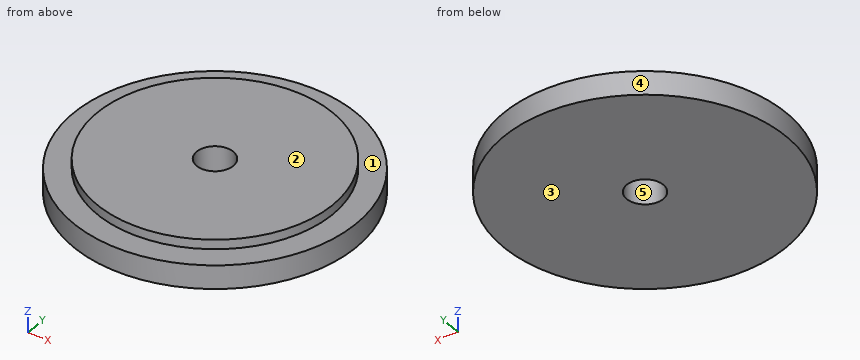
```python
from build123d import *

# Parameters (mm, degrees)
F0_R     = 15
F1_DEPTH = 2.5
F2_R     = 12.5
F3_DEPTH = 1
F4_R     = 1.94
F5_DEPTH = 3.5


with BuildPart() as f1:
    # F0 (on Top) → F1 (new body)
    with BuildSketch(Plane.XY):
        Circle(F0_R)
    extrude(amount=F1_DEPTH)

    # F2 (on face) → F3 (join)
    with BuildSketch(Plane.XY.offset(2.5)):
        Circle(F2_R)
    extrude(amount=F3_DEPTH)

    # F4 (on face) → F5 (cut, through all)
    with BuildSketch(Plane.XY.offset(3.5)):
        Circle(F4_R)
    extrude(amount=-F5_DEPTH, mode=Mode.SUBTRACT)


solid = f1.part
```
For this review, take the finished solid that the model builds, in its own axes (mm). Face numbers are marked on the shaded views. A direction names the side the tool comes from. Give positions to 0.01 mm unless a question says otherwise; leave off trailing zeros. Order: outer loops, then holes, each group sorted by start corner. A loop starts at its lowest first (then second) coordinate and runs counter-clockwise, first axis right, second up.
1) Take a section at D-D (z = 1.55). Give the boundary of the cut face in (x, y), then the cut area to 3 significant figures.
2) The part is to be moulded in two halves that separate along X. For the marked faces 3, 4 and 5, say which applies: released by +X, released by -X, zero draft, split by the parting line, or undercut.
3) Take a section at C-C (x = 12). Give the boundary of the cut face in (y, z).
4) Wall thickness on line 1 (Y direction, x = 0, z = 1.25); line 2 (X direction, y = -1, z = 2.45); line 3 (Z direction, x = 13.5, y = 3.5): over which ranges is each line inside the solid? List them lowest first.
5) For the marked faces 1 and 2, list the 3-axis set-ups (+Z, -Z, +X, -X, +Y, -Y) from which the entire face can be reached by the end or side of a thin tool; tool diameter is ignored.
6) Take a section at A-A (x = 0). Give the boundary of the cut face in (y, z), then the cut area to 3 significant figures.
Derived:
1. outline: circle Ø30 at (0, 0); hole circle Ø3.88 at (0, 0)
1. area: 695 mm2
2. face 3: zero draft
2. face 4: split by the parting line
2. face 5: undercut
3. outline: (-9, 0) - (9, 0) - (9, 2.5) - (3.5, 2.5) - (3.5, 3.5) - (-3.5, 3.5) - (-3.5, 2.5) - (-9, 2.5) - close
4. line 1: y = -15 to -1.94, 1.94 to 15
4. line 2: x = -14.97 to -1.66, 1.66 to 14.97
4. line 3: z = 0 to 2.5
5. face 1: +Z
5. face 2: +Z, +X, -X, +Y, -Y
6. outline: (-15, 0) - (-1.94, 0) - (-1.94, 3.5) - (-12.5, 3.5) - (-12.5, 2.5) - (-15, 2.5) - close; (1.94, 0) - (15, 0) - (15, 2.5) - (12.5, 2.5) - (12.5, 3.5) - (1.94, 3.5) - close
6. area: 86.4 mm2
